from build123d import *

# Parameters (mm, degrees)
BOSS_EXTRUDE1_DEPTH                              = 20
SKETCH4_R                                        = 17.5
CUT_EXTRUDE1_DEPTH                               = 11.453250926
SKETCH5_R                                        = 5
BOSS_EXTRUDE2_DEPTH                              = 10
CBORE_FOR_M5_HEX_HEAD_MACHINE_SCREW2_D           = 3.5
CBORE_FOR_M5_HEX_HEAD_MACHINE_SCREW2_DEPTH       = 11
CBORE_FOR_M5_HEX_HEAD_MACHINE_SCREW2_CBORE_D     = 7
CBORE_FOR_M5_HEX_HEAD_MACHINE_SCREW2_CBORE_DEPTH = 4
CBORE_FOR_M5_HEX_HEAD_MACHINE_SCREW2_TIP         = 1.75
CUT_EXTRUDE2_DEPTH                               = 65.71473925
CUT_EXTRUDE2_DEPTH_BACK                          = 65.71473925
SKETCH11_R                                       = 2.35


with BuildPart() as part:
    # Sketch2 → Boss-Extrude1 (new body)
    with BuildSketch(Plane.XY):
        with BuildLine():
            Line((42.376776125, 8.683218748), (-42.540089832, 8.683218747))
            add(Edge.make_bspline(
                [(-42.540089832, 8.683218747), (-61.647606257, -6.072667773), (-45.873698376, -22.15549797)],
                knots=[0, 0, 0, 1, 1, 1], degree=2))
            add(Edge.make_bspline(
                [(-45.873698376, -22.15549797), (0.203235462, -40.398996626), (45.873698397, -22.155497949)],
                knots=[0, 0, 0, 1, 1, 1], degree=2))
            add(Edge.make_bspline(
                [(45.873698397, -22.155497949), (61.713202875, -6.005950809), (42.376776125, 8.683218748)],
                knots=[0, 0, 0, 1, 1, 1], degree=2))
        make_face()
    extrude(amount=BOSS_EXTRUDE1_DEPTH)

    # Sketch4 → Cut-Extrude1 (cut)
    with BuildSketch(Plane.XY.offset(20)):
        with Locations((0, -11.063024907)):
            Circle(SKETCH4_R)
    extrude(amount=-CUT_EXTRUDE1_DEPTH, mode=Mode.SUBTRACT)

    # Sketch5 → Boss-Extrude2 (add)
    with BuildSketch(Plane.XY.offset(8.546749074)):
        with Locations((0, -11.063024907)):
            Circle(SKETCH5_R)
    extrude(amount=BOSS_EXTRUDE2_DEPTH)

    # CBORE for M5 Hex Head Machine Screw2
    with Locations(Plane(origin=(0, 0, 0), x_dir=(-1, 0, 0), z_dir=(0, 0, -1))):
        with Locations((-8.660254038, -6.129479586), (0, -21.129479586), (8.660254038, -6.129479586)):
            CounterBoreHole(CBORE_FOR_M5_HEX_HEAD_MACHINE_SCREW2_D / 2, CBORE_FOR_M5_HEX_HEAD_MACHINE_SCREW2_CBORE_D / 2, CBORE_FOR_M5_HEX_HEAD_MACHINE_SCREW2_CBORE_DEPTH, depth=CBORE_FOR_M5_HEX_HEAD_MACHINE_SCREW2_DEPTH)
            with Locations((0, 0, -(CBORE_FOR_M5_HEX_HEAD_MACHINE_SCREW2_DEPTH + CBORE_FOR_M5_HEX_HEAD_MACHINE_SCREW2_TIP / 2))):  # 90° drill point
                Cone(0, CBORE_FOR_M5_HEX_HEAD_MACHINE_SCREW2_D / 2, CBORE_FOR_M5_HEX_HEAD_MACHINE_SCREW2_TIP, mode=Mode.SUBTRACT)

    # Sketch11 → Cut-Extrude2 (cut, two sides: drawn at the far end of the back side and taken through both)
    with BuildSketch(Plane.XY.offset(20).offset(-CUT_EXTRUDE2_DEPTH_BACK)):
        with Locations((-34.669778537, -19.865188652)):
            Circle(SKETCH11_R)
        with Locations((-34.669778537, -7.616948648)):
            Circle(SKETCH11_R)
        with Locations((34.669778537, -7.616948648)):
            Circle(SKETCH11_R)
        with Locations((34.669778537, -19.865188652)):
            Circle(SKETCH11_R)
    extrude(amount=CUT_EXTRUDE2_DEPTH + CUT_EXTRUDE2_DEPTH_BACK, mode=Mode.SUBTRACT)


solid = part.part
Part model, mm, in its own coordinate system. A direction names the side the tool comes from. Coordinates: 2 decimals unless noted, no trailing zeros. Write each question's results on one line, items separated by ' | '. Start each with the question number.
Q1. Drop flat-ended pins along their axis: pin 1 Ø3 at (x, y) = (-0.5, -11.5) entering from +Z; pin 2 Ø5.5 at (x, y) = (0, -21.13) entering from +Z; pin 3 Ø2 at (x, y) = (-9.5, -7) entering from -Z; pin 4 Ø4 at (x, y) = (34.67, -7.62) entering from +Z. Give the stop position or say it passes through.
Q2. Two-plate mould, pull along X, no slides. Class faces 4 (the flat face through (-15, 1, 20)), 5 (the cylindrical face through (9.419, -9.546, 1.972)): +X half, -X half, draft (parallel to the pull), parting line (faces both ways), or undercut.
Q3. Slice it at A-A on x = -35. Give the number of separate pieces and of enclosed holes in the cut face, and give its area (3 significant figures).
Q4. Which spindle directions (+Z, -Z, +X, -X, +Y, -Y) get a long thin tool onto all of the face, cutting with end or side? Do faces 1 (the flat face through (4, -15, 8.547)), 2 (the cylindrical face through (-1.882, -18.178, 1.972)), 3 (the cylindrical face through (35.754, -9.702, 9.86)). Say none if no direction does.
Q5. Probe line 1 along Y through (x, z) = (0, 10.25); line 2 along Y through (x, z) = (33.5, 18.25); line 3 along X through (y, z) = (-6, 6.75). List the from-to ranges inside material, lowest first.
Answer:
1) pin 1: stops at z = 18.55 | pin 2: stops at z = 8.55 | pin 3: stops at z = 4 | pin 4: passes through
2) face 4: draft | face 5: undercut
3) separate pieces: 3 | enclosed holes: 0 | area: 507 mm2
4) face 1: +Z | face 2: -Z | face 3: +Z, -Z
5) line 1: y = -31.28 to -28.56, -16.06 to -6.06, 6.44 to 8.68 | line 2: y = -26.43 to -21.9, -17.83 to -9.66, -5.58 to 8.68 | line 3: x = -52.88 to -36.38, -32.96 to -10.41, -6.92 to 6.92, 10.41 to 32.96, 36.38 to 52.87
